Autodesk Inventor part; units mm, degrees
ref_plane "YZ Plane" through (0, 0, 0) normal (1, 0, 0) x (0, 1, 0)
ref_plane "XZ Plane" through (0, 0, 0) normal (0, 1, 0) x (-1, 0, 0)
ref_plane "XY Plane" through (0, 0, 0) normal (0, 0, 1) x (1, 0, 0)
sketch "Náčrt2" plane through (0, 0, 0) normal (0, 0, 1) x (1, 0, 0)
  line L0 (0, 0) -> (190, 0)
  line L1 (190, 0) -> (190, -45)
  line L2 (190, -45) -> (0, -45)
  line L3 (0, -45) -> (0, 0)
  dimension "d2" = 190
  dimension "d3" = 45
extrude "Vysunutí2" add sketch "Náčrt2" along normal blind 4
sketch "Náčrt3" plane through (0, 0, 4) normal (0, 0, 1) x (1, 0, 0)
  line L0 (190, 0) -> (0, 0)
  line L1 (0, -45) -> (190, -45)
  line L2 (190, -45) -> (190, 0)
  line L3 (190, 0) -> (0, 0)
  line L4 (0, 0) -> (0, -45)
  line L5 (4, -41) -> (186, -41)
  line L6 (186, -41) -> (186, -4)
  line L7 (186, -4) -> (4, -4)
  line L8 (4, -4) -> (4, -41)
  dimension "d7" = 4
extrude "Vysunutí3" add sketch "Náčrt3" along normal blind 120
sketch "Náčrt4" plane through (0, -45, 0) normal (0, -1, 0) x (1, 0, 0)
  line L0 (4, 124) -> (186, 124)
  line L1 (182, 124) -> (58, 124)
  line L2 (58, 124) -> (58, 24)
  line L3 (58, 24) -> (182, 24)
  line L4 (182, 24) -> (182, 124)
  line L5 (190, 0) -> (190, 124)
  point P0 (0, 0)
  dimension "d10" = 8
  dimension "d11" = 100
  dimension "d12" = 124
extrude "Vysunutí4" cut sketch "Náčrt4" against normal blind 10
sketch "Náčrt6" plane through (4, -41, 4) normal (0, 1, 0) x (1, 0, 0)
  line L0 (-4, 4) -> (186, 4)
  line L1 (-4, 4) -> (-4, -120)
  line L2 (178, -120) -> (178, -20)
  line L3 (178, -20) -> (54, -20)
  line L4 (54, -20) -> (54, -120)
  line L5 (-4, -120) -> (54, -120)
  line L6 (-4, 4) -> (-4, -120)
  line L7 (-4, 4) -> (186, 4)
  line L8 (186, 4) -> (186, -120)
  line L9 (178, -120) -> (186, -120)
extrude "Vysunutí6" add sketch "Náčrt6" along normal blind 3
sketch "Náčrt7" plane through (0, 0, 124) normal (0, 0, 1) x (1, 0, 0)
  line L0 (184.5, -42) -> (4, -42)
  line L1 (4, -42) -> (4, -40)
  line L2 (4, -40) -> (184.5, -40)
  line L3 (184.5, -40) -> (184.5, -42)
  line L4 (182, -38) -> (182, -45)
  line L5 (182, -45) -> (190, -45)
  point P0 (0, 0)
  dimension "d25" = 2.5
  dimension "d26" = 2
  dimension "d27" = 3
  dimension "d28" = 180.5
extrude "Vysunutí7" cut sketch "Náčrt7" against normal blind 105
sketch "Náčrt8" plane through (4, -38, 4) normal (0, 1, 0) x (1, 0, 0)
  line L0 (54, -120) -> (54, -20)
  line L1 (0, -120) -> (54, -120)
  line L2 (54, -120) -> (0, -120)
  line L3 (0, -120) -> (0, -20)
  line L4 (0, -20) -> (54, -20)
  line L5 (54, -20) -> (54, -120)
  point P0 (-4, 4)
  point P1 (54, -20)
  dimension "d31" = 54
  dimension "d32" = 100
extrude "Vysunutí8" cut sketch "Náčrt8" against normal up to surface (4 mm away)
sketch "Náčrt9" plane through (4, -38, 4) normal (0, 1, 0) x (1, 0, 0)
  line L0 (54, -20) -> (54, -120)
  line L1 (0, 40) -> (54, 40)
  line L2 (54, 40) -> (54, -20)
  line L3 (54, -20) -> (0, -20)
  line L4 (0, -20) -> (0, 40)
  point P0 (-4, 4)
  dimension "d35" = 54
extrude "Vysunutí9" cut sketch "Náčrt9" against normal blind 4
sketch "Náčrt10" plane through (190, -45, 0) normal (1, 0, 0) x (0, 0, -1)
  circle A0 centre (-109, 25) radius 2.5
  line L0 (0, 0) -> (-124, 0)
  line L1 (-124, 0) -> (-124, 45)
  point P0 (0, 45)
  dimension "d38" = 5
  dimension "d39" = 25
  dimension "d40" = 15
extrude "Vysunutí10" cut sketch "Náčrt10" against normal through all
sketch "Náčrt11" plane through (0, 0, 4) normal (0, 0, 1) x (1, 0, 0)
  circle A0 centre (25.2842, -14.6015) radius 2.5
  circle A1 centre (35.2842, -14.6015) radius 2.5
  circle A2 centre (45.2842, -14.6015) radius 2.5
  circle A3 centre (31.1056, -24.6015) radius 2.5
  circle A4 centre (41.1056, -24.6015) radius 2.5
  circle A5 centre (36.7049, -34.6015) radius 2.5
  line L0 (25.2842, -14.6015) -> (59.2692, -14.6015) construction
  line L1 (31.1056, -24.6015) -> (52.5835, -24.6015) construction
  point P0 (0, 0)
  dimension "d43" = 5
  dimension "d44" = 5
  dimension "d45" = 5
  dimension "d46" = 5
  dimension "d47" = 5
  dimension "d48" = 5
  dimension "d49" = 10
  dimension "d50" = 10
  dimension "d51" = 10
  dimension "d52" = 10
  dimension "d53" = 10
extrude "Vysunutí11" cut sketch "Náčrt11" against normal through all
pattern_linear "Obdélníkové pole1" count 3 spacing 55 along (1, 0, 0) of "Vysunutí11"
sketch "Náčrt12" plane through (0, 0, 0) normal (0, 0, -1) x (-1, 0, 0)
  line L0 (-4, -42) -> (-58, -42)
  line L1 (-58, -38) -> (-4, -38)
  line L2 (-58, -42) -> (-58, -38)
  line L3 (-4, -38) -> (-4, -42)
  point P0 (0, 0)
extrude "Vysunutí12" add sketch "Náčrt12" against normal up to surface (4 mm away)
sketch "Náčrt13" plane through (190, -45, 0) normal (1, 0, 0) x (0, 0, -1)
  line L0 (-20, 12) -> (-20, 37) construction
  line L1 (-15, 17) -> (-15, 32)
  line L2 (-25, 32) -> (-25, 17)
  arc A0 (-25, 17) -> (-15, 17) centre (-20, 17) ccw
  arc A1 (-15, 32) -> (-25, 32) centre (-20, 32) ccw
  line L3 (0, 45) -> (-124, 45)
  line L4 (0, 0) -> (0, 45)
  point P0 (-20, 24.5)
  dimension "d61" = 25
  dimension "d62" = 10
  dimension "d63" = 8
  dimension "d64" = 20
extrude "Vysunutí13" cut sketch "Náčrt13" against normal through all
sketch "Náčrt14" plane through (0, 0, 0) normal (0, 1, 0) x (1, 0, 0)
  line L0 (190, 0) -> (190, -124)
  line L1 (190, -60) -> (210, -60)
  line L2 (210, -60) -> (210, -40)
  line L3 (210, -40) -> (190, -40)
  line L4 (190, -40) -> (190, -60)
  line L5 (190, 0) -> (0, 0)
  line L6 (190, 0) -> (195, 0)
  line L7 (195, 0) -> (210, -40)
  circle A0 centre (200, -50) radius 2.5
  line L8 (4, -124) -> (186, -124)
  line L9 (95, -124) -> (95, 0) construction
  line L10 (0, 0) -> (0, -124)
  line L11 (0, -60) -> (-20, -60)
  line L12 (-20, -60) -> (-20, -40)
  line L13 (-20, -40) -> (0, -40)
  line L14 (0, 0) -> (190, 0)
  line L15 (0, 0) -> (-5, 0)
  line L16 (-5, 0) -> (-20, -40)
  circle A1 centre (-10, -50) radius 2.5
  dimension "d67" = 20
  dimension "d68" = 20
  dimension "d69" = 40
  dimension "d70" = 5
  dimension "d71" = 5
  dimension "d72" = 10
  dimension "d73" = 10
extrude "Vysunutí14" add sketch "Náčrt14" against normal blind 4
properties part number "krab2-ver1" material "11 500"
Could you check a few things on this model? Use its own coordinates, in mm. A direction names the side the tool comes from. Give positions to 0.01 mm unless a question says otherwise; leave off trailing zeros. Order: outer loops, then holes, each group sorted by start corner. A loop starts at its lowest first (then second) coordinate and runs counter-clockwise, first axis right, second up.
1. I need wall thicknesses on L1, parallel to X at y = -8.5, z = 92; L2, parallel to Y at x = 11, z = 116.5; L3, parallel to Y at x = 174.5, z = 57.5. Which ranges of each line are inside material? Lowest first, please.
2. We'd pull the mould along Z, two halves only. Please class faces 5 (the flat face through (0, -23, 61)), 6 (the cylindrical face through (-10.54, -1.97, 52.44)), 7 (the flat face through (200, -2, 60)): pulls with the +Z half, pulls with the -Z half, needs draft (parallel to the pull), parting line crosses it, or undercut.
3. Suppose I cut it at C-C (z = 85.5). List the corners of the cut face in (x, y) for me, plus the area to 3 significant figures.
4. Suppose I cut it at A-A (z = 50). List the corners of the cut face in (x, y) for me.
5. Suppose I cut it at B-B (x = 9). List the corners of the cut face in (y, z) for me.
6. Will these pins go through, and if not, where does the flat tip stop? P1, Ø6, axis at x = 197, z = 31, coming from the -Y side; P2, Ø6.5, axis at x = 155.28, y = -14.6, coming from the +Z side; P3, Ø6, axis at x = 128, y = -5.5, coming from the +Z side; P4, Ø0.6, axis at x = 137, y = -41.5, coming from the +Z side.
7. For faces 1 (the flat face through (198, -4, 36)), 2 (the flat face through (-8, -4, 36)), 3 (the flat face through (58, -40, 14)), 4 (the flat face through (188, -20, 25)), which set-ups out of +Z, -Z, +X, -X, +Y, -Y let a thin tool reach every point of the face, with its end or its side?
Solved:
1. L1: x = 0 to 4, 186 to 190
1. L2: y = -45 to -42, -4 to 0
1. L3: y = -4 to 0
2. face 5: needs draft
2. face 6: undercut
2. face 7: pulls with the +Z half
3. outline: (0, -45) - (58, -45) - (58, -42) - (4, -42) - (4, -4) - (186, -4) - (186, -38) - (182, -38) - (182, -40) - (184.5, -40) - (184.5, -42) - (182, -42) - (182, -45) - (190, -45) - (190, 0) - (0, 0) - close
3. area: 1,270 mm2
4. outline: (-20, -4) - (-12.5, -4) - (-12.5, 0) - (-20, 0) - close; (-7.5, -4) - (0, -4) - (0, -45) - (58, -45) - (58, -42) - (4, -42) - (4, -4) - (186, -4) - (186, -38) - (182, -38) - (182, -40) - (184.5, -40) - (184.5, -42) - (182, -42) - (182, -45) - (190, -45) - (190, -4) - (197.5, -4) - (197.5, 0) - (-7.5, 0) - close; (202.5, -4) - (210, -4) - (210, 0) - (202.5, 0) - close
5. outline: (-45, 0) - (0, 0) - (0, 124) - (-4, 124) - (-4, 4) - (-42, 4) - (-42, 124) - (-45, 124) - close
6. P1: stops at y = -4
6. P2: stops at z = 4
6. P3: stops at z = 124
6. P4: stops at z = 19
7. face 1: +Z, -Z, +X, -Y
7. face 2: +Z, -Z, -X, -Y
7. face 3: +Z
7. face 4: +X, -X
